Geometry: final body of the model. Coordinates: model frame, mm. A direction names the side the tool comes from. Coordinates: 2 decimals unless noted, no trailing zeros. Order: outer loops, then holes, each group sorted by start corner. A loop starts at its lowest first (then second) coordinate and runs counter-clockwise, first axis right, second up. Notation, with made-up numbers: M 28.25,-1.75 L 79.25,-1.75 A30 cw 79.25,30.25 Z; hole C 76.5,35 d5. An arc over 180 degrees is marked long. Write item = value, one per line. Start each with the question number.
```python
from build123d import *

# Parameters (mm, degrees)
SKETCH1_W                = 12.7
SKETCH1_H                = 12.7
BOSS_EXTRUDE1_DEPTH      = 1.27
SKETCH2_R                = 1.211003997
SKETCH2_R_2              = 1.271770102
SKETCH2_R_3              = 1.338907355
SKETCH2_R_4              = 1.365975295
CUT_EXTRUDE1_DEPTH       = 1.27
SKETCH3_R                = 3.438076728
BOSS_EXTRUDE2_DEPTH      = 1.778
BOSS_EXTRUDE3_DEPTH      = 3.048
BOSS_EXTRUDE3_DEPTH_BACK = 2.54
SKETCH4_R                = 1.176424435


with BuildPart() as part:
    # Sketch1 → Boss-Extrude1 (new body)
    with BuildSketch(Plane(origin=(0, 0, 0), x_dir=(1, 0, 0), z_dir=(0, 1, 0))):
        with Locations((61.354700157, 8.680443435)):
            Rectangle(SKETCH1_W, SKETCH1_H)
    extrude(amount=BOSS_EXTRUDE1_DEPTH)

    # Sketch2 → Cut-Extrude1 (cut)
    with BuildSketch(Plane(origin=(0, 1.27, 0), x_dir=(1, 0, 0), z_dir=(0, 1, 0))):
        with Locations(Location((56.671293602, 13.271817518, 0), (0, 0, 270))):
            Circle(SKETCH2_R)
        with Locations(Location((65.762094704, 13.177612325, 0), (0, 0, 270))):
            Circle(SKETCH2_R_2)
        with Locations(Location((56.812601392, 4.039708628, 0), (0, 0, 270))):
            Circle(SKETCH2_R_3)
        with Locations(Location((65.667889511, 4.086811224, 0), (0, 0, 270))):
            Circle(SKETCH2_R_4)
    extrude(amount=-CUT_EXTRUDE1_DEPTH, mode=Mode.SUBTRACT)

    # Sketch3 → Boss-Extrude2 (add)
    with BuildSketch(Plane(origin=(0, 1.27, 0), x_dir=(1, 0, 0), z_dir=(0, 1, 0))):
        with Locations(Location((61.153985379, 8.608321241, 0), (0, 0, 90))):
            Circle(SKETCH3_R)
    extrude(amount=BOSS_EXTRUDE2_DEPTH)

    # Sketch4 → Boss-Extrude3 (add, two sides: drawn at the far end of the back side and taken through both)
    with BuildSketch(Plane(origin=(0, 3.048, 0), x_dir=(1, 0, 0), z_dir=(0, 1, 0)).offset(-BOSS_EXTRUDE3_DEPTH_BACK)):
        with Locations(Location((61.122804521, 8.49685939, 0), (0, 0, 270))):
            Circle(SKETCH4_R)
    extrude(amount=BOSS_EXTRUDE3_DEPTH + BOSS_EXTRUDE3_DEPTH_BACK)


solid = part.part
```
Item 1: Section query B-B on z = -4.5. Output: boundary loops of the cut face in (x, y).
Item 2: Draft query along X for faces 3 (the cylindrical face through (60.7, 4.6, -7.4)), 4 (the cylindrical face through (64.334, 0.644, -4.383)), 5 (the flat face through (63, 3.048, -9)). Return one class per face: pulls with the +X half, pulls with the -X half, needs draft (parallel to the pull), parting line crosses it, or undercut.
Item 3: Reachability of faces 1 (the cylindrical face through (55.6, 0.64, -12.71)), 2 (the cylindrical face through (58.8, 2.1, -6.1)) from +Z, -Z, +X, -X, +Y, -Y: full face, straight path, thin tool, end or side. Return the list, or none.
Item 4: Section query D-D on z = -10.25. Output: boundary loops of the cut face in (x, y).
Item 5: Material intervals for probe 1 along Z at (x, y) = (66, 0.75); probe 2 along X at (y, z) = (0.5, -3.75); probe 3 along Y at (x, z) = (64, -3), sorted ascending. Write a range as [from, to].
Item 6: Section query A-A on x = 56.5. Output: boundary loops of the cut face in (y, z), and give its area (3 significant figures).
Item 7: First-contact query: pin 1 (3 mm diameter, centred on x = 58.5, y = 3.5, fed in from -Z); pin 2 (2 mm diameter, centred on x = 65, z = -11, fed in from +Y). Flat tips, straight axial feed; report the tip coordinate or a pass-through.
Item 8: Section query C-C on y = 1. Output: boundary loops of the cut face in (x, z), and give its area (3 significant figures).
Ans:
q1.outline = M 55,0 L 55.56,0 L 55.56,1.27 L 55,1.27 Z; M 58.07,0 L 64.37,0 L 64.37,1.27 L 58.07,1.27 Z; M 66.97,0 L 67.7,0 L 67.7,1.27 L 66.97,1.27 Z
q2.face_3 = parting line crosses it
q2.face_4 = undercut
q2.face_5 = needs draft
q3.face_1 = +Y, -Y
q3.face_2 = +Y
q4.outline = M 55,0 L 67.7,0 L 67.7,1.27 L 64.17,1.27 L 64.17,3.05 L 58.13,3.05 L 58.13,1.27 L 55,1.27 Z
q5.probe_1 = [-15.03, -14.43], [-11.93, -5.41], [-2.76, -2.33]
q5.probe_2 = [55, 55.51], [58.12, 64.34], [66.99, 67.7]
q5.probe_3 = [0, 1.27]
q6.outline = M 0,-15.03 L 1.27,-15.03 L 1.27,-14.47 L 0,-14.47 Z; M 0,-12.07 L 1.27,-12.07 L 1.27,-5.34 L 0,-5.34 Z; M 0,-2.74 L 1.27,-2.74 L 1.27,-2.33 L 0,-2.33 Z
q6.area = 9.78 mm^2
q7.pin_1 = -11.82
q7.pin_2 = 1.27
q8.outline = M 55,-15.03 L 67.7,-15.03 L 67.7,-2.33 L 55,-2.33 Z; hole C 56.67,-13.27 d2.42; hole C 56.81,-4.04 d2.68; hole C 65.67,-4.09 d2.73; hole C 65.76,-13.18 d2.54
q8.area = 140 mm^2
